Input: dimensioned drawing with shaded views. Units: mm. Origin: part minimum x, y, z. Round coordinates to 2 decimals unless told otherwise and drop trailing zeros. Loops run counter-clockwise (first coordinate to the right, second up) from the corner with the lowest first, then second, coordinate; pieces in that order, holes last.
Item 1: Ray query, L1, parallel to X at y = 5, z = 1.7 (1 decimal); L2, parallel to Y at x = 10, z = 2.55 (1 decimal); L3, parallel to Y at x = 20, z = 1.5 (1 decimal). Return the intervals inside material, ascending.
Item 2: First-contact query: P1, Ø1, axis at y = 21, z = 1.5, coming from the -X side; P2, Ø2, axis at y = 5.5, z = 2, coming from the +X side; P3, Ø2, axis at x = 11, z = 1.5, coming from the +Y side. Flat tips, straight axial feed; report the tip coordinate or a pass-through.
Item 3: Section query A-A on z = 0.85. Return loops of the section in (x, y), then the cut area to 3 significant figures.
Item 4: Pull-direction query (Y, two-part tool) for the marked faces 1, 2 and 3; classes: released by +Y, released by -Y, zero draft, split by the parting line, or undercut.
Item 5: Section query B-B on x = 18.5. Give the number of separate pieces and of enclosed holes in the cut face.
Item 6: Section query D-D on z = 3.05. Return loops of the section in (x, y), then the cut area to 3 significant figures.
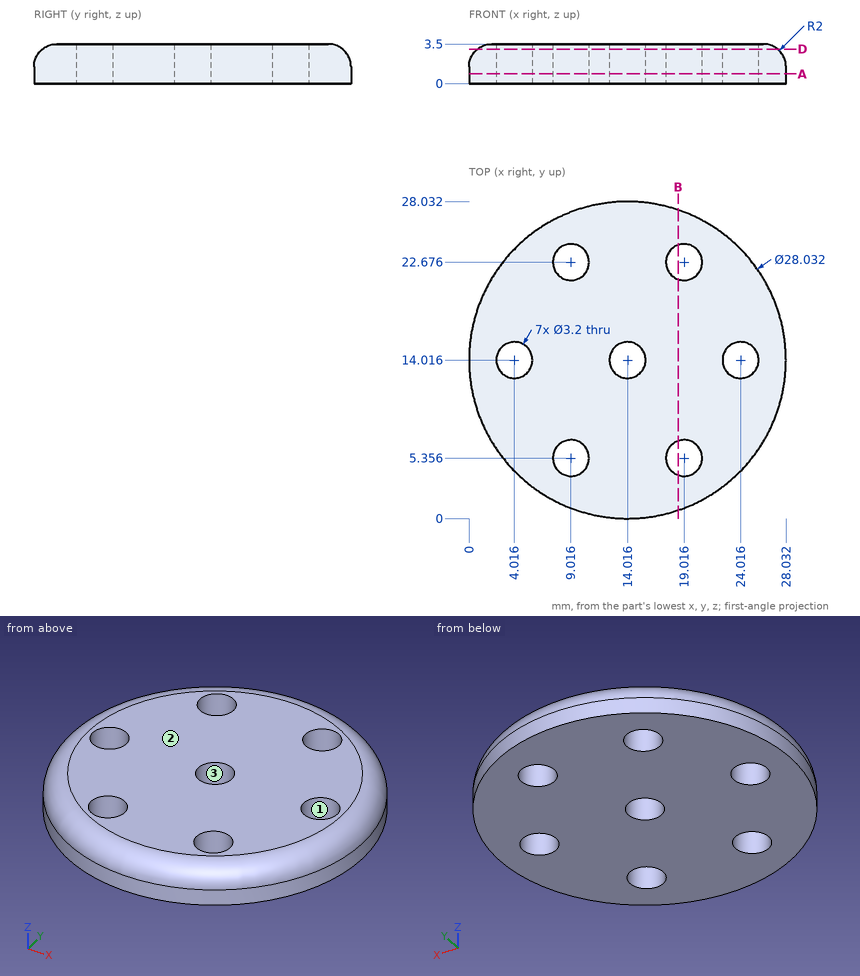
Data:
1. L1: x = 3.3 to 7.5, 10.6 to 17.5, 20.6 to 24.7
1. L2: y = 0.9 to 4.1, 6.6 to 21.4, 23.9 to 27.1
1. L3: y = 1.3 to 4.1, 6.6 to 21.4, 23.9 to 26.7
2. P1: stops at x = 1.59
2. P2: stops at x = 25.81
2. P3: stops at y = 27.89
3. outline: circle Ø28.03 at (14.02, 14.02); hole circle Ø3.2 at (4.02, 14.02); hole circle Ø3.2 at (9.02, 5.36); hole circle Ø3.2 at (9.02, 22.68); hole circle Ø3.2 at (14.02, 14.02); hole circle Ø3.2 at (19.02, 5.36); hole circle Ø3.2 at (19.02, 22.68); hole circle Ø3.2 at (24.02, 14.02)
3. area: 561 mm2
4. face 1: undercut
4. face 2: zero draft
4. face 3: undercut
5. separate pieces: 3
5. enclosed holes: 0
6. outline: circle Ø26.56 at (14.02, 14.02); hole circle Ø3.2 at (4.02, 14.02); hole circle Ø3.2 at (9.02, 5.36); hole circle Ø3.2 at (9.02, 22.68); hole circle Ø3.2 at (14.02, 14.02); hole circle Ø3.2 at (19.02, 5.36); hole circle Ø3.2 at (19.02, 22.68); hole circle Ø3.2 at (24.02, 14.02)
6. area: 498 mm2
